Check sheet for the modelled part. Datum: model origin and axes. Units: mm. A direction names the side the tool comes from. Round coordinates to 2 decimals unless told otherwise and drop trailing zeros. Order: outer loops, then holes, each group sorted by start corner. A loop starts at its lowest first (then second) coordinate and runs counter-clockwise, first axis right, second up. Notation, with made-up numbers: (52, -32) -> (62, -32) arc R19 cw to (62, -23) -> close; hole circle Ø11 at (85.25, 75.25). An arc over 180 degrees is marked (long way). Answer in a Markdown table with one row per item. Add a question column.
1. Sectioned sample at C-C, the plane z = -6.5. Record the boundary of the cut face in (x, y), then the cut area to 3 significant figures.
2. Sectioned sample at D-D, the plane y = -6.5. Record the boundary of the cut face in (x, z), then the cut area to 3 significant figures.
3. Draft check along Y on faces 4 (the flat face through (-1, 0, -12.5)), 5 (the flat face through (-46, -2.5, 0)), 6 (the cylindrical face through (57.605, 7.852, 7.974)). Enter one of: +Y half, -Y half, draft (parallel to the pull), parting line (faces both ways), or undercut.
4. Material ranges on L1, parallel to Y at x = 55.75, z = -6.5; L2, parallel to X at y = 10, z = 5.75, recorded low to high. Write a range as from..to.
5. Depth check by flat-ended pin: P1, Ø3, axis at x = -45, z = 0.5, coming from the +Y side; P2, Ø1.5, axis at x = 38.5, y = -4.5, coming from the +Z side; P3, Ø2, axis at y = 6.5, z = 6.5, coming from the -X side; P4, Ø3.5, axis at y = -6.5, z = 6.5, coming from the +X side. Enter the tip coordinate at first touch or a pass-through.
6. Sectioned sample at A-A, the plane z = 6.5. Record the boundary of the cut face in (x, y), then the cut area to 3 significant figures.
7. Access from +Z, -Z, +X, -X, +Y, -Y to the whole of each face (thin tool, end or side, straight path). Record for faces 1 (the flat face through (50, -6, -6)), 2 (the flat face through (-50, 6, -7)), 3 (the cylindrical face through (-2, 5, 0)).
8. Sectioned sample at B-B, the plane x = 53. Record the boundary of the cut face in (y, z).
```python
from build123d import *

# Parameters (mm, degrees)
BOSS_EXTRUDE1_DEPTH = 12.5
SKETCH2_R           = 2
CUT_EXTRUDE1_DEPTH  = 15
SKETCH3_R           = 2
CUT_EXTRUDE2_DEPTH  = 15


with BuildPart() as part:
    # Sketch1 → Boss-Extrude1 (new, symmetric)
    with BuildSketch(Plane(origin=(0, 0, 0), x_dir=(1, 0, 0), z_dir=(0, 1, 0))):
        Polygon((-65, 12.5), (65, 12.5), (65, -12.5), (40, -12.5), (40, 0.5), (37, 0.5), (37, -12.5), (-37, -12.5), (-37, 0.5), (-40, 0.5), (-40, -12.5), (-65, -12.5), align=None)
    extrude(amount=BOSS_EXTRUDE1_DEPTH, both=True)

    # Sketch2 → Cut-Extrude1 (cut)
    with BuildSketch(Plane(origin=(65, 0, 0), x_dir=(0, 0, -1), z_dir=(1, 0, 0))):
        with Locations((-6.5, 6.5)):
            Circle(SKETCH2_R)
        with Locations(Location((6.5, 6.5, 0), (0, 0, 180))):
            Circle(SKETCH2_R)
        with Locations((6.5, -6.5)):
            Circle(SKETCH2_R)
        with Locations(Location((-6.5, -6.5, 0), (0, 0, 180))):
            Circle(SKETCH2_R)
    cut_extrude1 = extrude(amount=-CUT_EXTRUDE1_DEPTH, mode=Mode.SUBTRACT)

    # Sketch3 → Cut-Extrude2 (cut)
    with BuildSketch(Plane(origin=(0, 12.5, 0), x_dir=(1, 0, 0), z_dir=(0, 1, 0))):
        with Locations(Location((46, 0, 0), (0, 0, 270))):
            Circle(SKETCH3_R)
        with Locations(Location((0, 0, 0), (0, 0, 270))):
            Circle(SKETCH3_R)
        with Locations(Location((-46, 0, 0), (0, 0, 270))):
            Circle(SKETCH3_R)
    extrude(amount=-CUT_EXTRUDE2_DEPTH, mode=Mode.SUBTRACT)

    # Mirror1: Cut-Extrude1 across plane
    add(cut_extrude1.mirror(Plane(origin=(0, 0, 0), x_dir=(0, 0, 1), z_dir=(1, 0, 0))), mode=Mode.SUBTRACT)


solid = part.part
```
Answer key:
| question | item | result |
|---|---|---|
| 1 | outline | (-65, -12.5) -> (65, -12.5) -> (65, -8.5) -> (50, -8.5) -> (50, -4.5) -> (65, -4.5) -> (65, 4.5) -> (50, 4.5) -> (50, 8.5) -> (65, 8.5) -> (65, 12.5) -> (-65, 12.5) -> (-65, 8.5) -> (-50, 8.5) -> (-50, 4.5) -> (-65, 4.5) -> (-65, -4.5) -> (-50, -4.5) -> (-50, -8.5) -> (-65, -8.5) -> close |
| 1 | area | 3,010 mm² |
| 2 | outline | (-65, -12.5) -> (65, -12.5) -> (65, -8.5) -> (50, -8.5) -> (50, -4.5) -> (65, -4.5) -> (65, 4.5) -> (50, 4.5) -> (50, 8.5) -> (65, 8.5) -> (65, 12.5) -> (40, 12.5) -> (40, -0.5) -> (37, -0.5) -> (37, 12.5) -> (-37, 12.5) -> (-37, -0.5) -> (-40, -0.5) -> (-40, 12.5) -> (-65, 12.5) -> (-65, 8.5) -> (-50, 8.5) -> (-50, 4.5) -> (-65, 4.5) -> (-65, -4.5) -> (-50, -4.5) -> (-50, -8.5) -> (-65, -8.5) -> close |
| 2 | area | 2,930 mm² |
| 3 | face 4 | draft |
| 3 | face 5 | +Y half |
| 3 | face 6 | undercut |
| 4 | L1 | y = -12.5..-8.5, -4.5..4.5, 8.5..12.5 |
| 4 | L2 | x = -65..-40, -37..37, 40..65 |
| 5 | P1 | stops at y = 12.5 |
| 5 | P2 | stops at z = -0.5 |
| 5 | P3 | stops at x = -50 |
| 5 | P4 | stops at x = 50 |
| 6 | outline | (-65, -12.5) -> (-40, -12.5) -> (-40, 12.5) -> (-65, 12.5) -> (-65, 8.5) -> (-50, 8.5) -> (-50, 4.5) -> (-65, 4.5) -> (-65, -4.5) -> (-50, -4.5) -> (-50, -8.5) -> (-65, -8.5) -> close; (-37, -12.5) -> (37, -12.5) -> (37, 12.5) -> (-37, 12.5) -> close; (40, -12.5) -> (65, -12.5) -> (65, -8.5) -> (50, -8.5) -> (50, -4.5) -> (65, -4.5) -> (65, 4.5) -> (50, 4.5) -> (50, 8.5) -> (65, 8.5) -> (65, 12.5) -> (40, 12.5) -> close |
| 6 | area | 2,860 mm² |
| 7 | face 1 | +X |
| 7 | face 2 | -X |
| 7 | face 3 | +Y |
| 8 | outline | (-12.5, -12.5) -> (12.5, -12.5) -> (12.5, 12.5) -> (-12.5, 12.5) -> close; hole circle Ø4 at (-6.5, -6.5); hole circle Ø4 at (-6.5, 6.5); hole circle Ø4 at (6.5, -6.5); hole circle Ø4 at (6.5, 6.5) |
